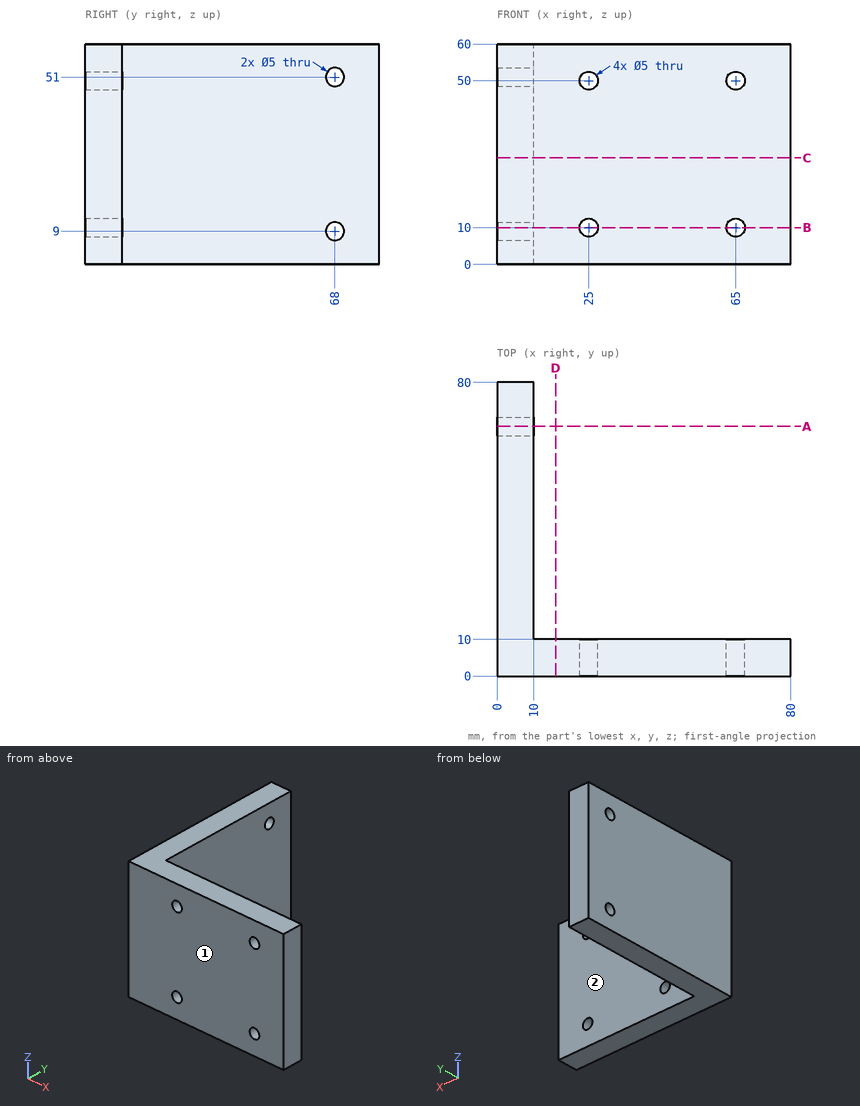
The figure shows three views and two pictorial views of one solid part (mm, origin at its lowest corner). Answer the questions. A direction names the side the tool comes from. Give positions to 0.01 mm unless a question says otherwise; leave off trailing zeros. Order: outer loops, then holes, each group sorted by start corner. A loop starts at its lowest first (then second) coordinate and runs counter-clockwise, first axis right, second up. Notation, with made-up numbers: (37.25, 64.25) -> (95.25, 64.25) arc R31 ccw to (95.25, 101.25) -> close; hole circle Ø8 at (48.5, 60.25). An arc over 180 degrees is marked (long way). Answer as CSV lines item,"result". Start each with the question number.
Q1. A cutting plane is placed at D-D (x = 16). Determine the outline of the cut face in (y, z).
Q2. Given pin 1 (2 mm diameter, centred on x = 49.5, z = 49.5, fed in from +Y); pin 2 (8 mm diameter, centred on y = 43, z = 41, fed in from +X), each flat-ended and moving along its own axis, determine where each tip first touches the part or whether it passes through.
Q3. Find the intervals of material crossed by L1, parallel to X at y = 7, z = 50; L2, parallel to Z at x = 3.5, y = 68; L3, parallel to Y at x = 8.25, z = 9, in increasing order.
Q4. Which of the six approach directions +Z, -Z, +X, -X, +Y, -Y give full straight-line access (tool end or side, diameter ignored) to the marked faces 1 and 2?
Q5. A cutting plane is placed at A-A (y = 68). Determine the outline of the cut face in (x, z).
Q6. A cutting plane is placed at B-B (z = 10). Determine the outline of the cut face in (x, y).
Q7. A cutting plane is placed at C-C (z = 29). Determine the outline of the cut face in (x, y).
Results found:
1,outline,"(0, 0) -> (10, 0) -> (10, 60) -> (0, 60) -> close"
2,pin 1,"y = 10"
2,pin 2,"x = 10"
3,L1,"0 to 22.5, 27.5 to 62.5, 67.5 to 80"
3,L2,"0 to 6.5, 11.5 to 48.5, 53.5 to 60"
3,L3,"0 to 65.5, 70.5 to 80"
4,face 1,"+Z, -Z, +X, -X, -Y"
4,face 2,"+Z, -Z, +X, +Y"
5,outline,"(0, 0) -> (10, 0) -> (10, 6.5) -> (0, 6.5) -> close; (0, 11.5) -> (10, 11.5) -> (10, 48.5) -> (0, 48.5) -> close; (0, 53.5) -> (10, 53.5) -> (10, 60) -> (0, 60) -> close"
6,outline,"(0, 0) -> (22.5, 0) -> (22.5, 10) -> (10, 10) -> (10, 65.71) -> (0, 65.71) -> close; (0, 70.29) -> (10, 70.29) -> (10, 80) -> (0, 80) -> close; (27.5, 0) -> (62.5, 0) -> (62.5, 10) -> (27.5, 10) -> close; (67.5, 0) -> (80, 0) -> (80, 10) -> (67.5, 10) -> close"
7,outline,"(0, 0) -> (80, 0) -> (80, 10) -> (10, 10) -> (10, 80) -> (0, 80) -> close"
